Study the drawing (mm; zero at the part's minimum x, y, z) and answer. Give positions to 0.01 mm unless a question says otherwise; leave off trailing zeros. Loops run counter-clockwise (first coordinate to the right, second up) from the corner with the lowest first, then second, coordinate; pieces in that order, holes last. Notation, with made-up numbers: M 26,83.25 L 36,83.25 A13 ccw 36,107.25 Z; hole C 5,26 d6. An arc over 180 degrees is marked long. Return JSON: item names as keys, results as strings.
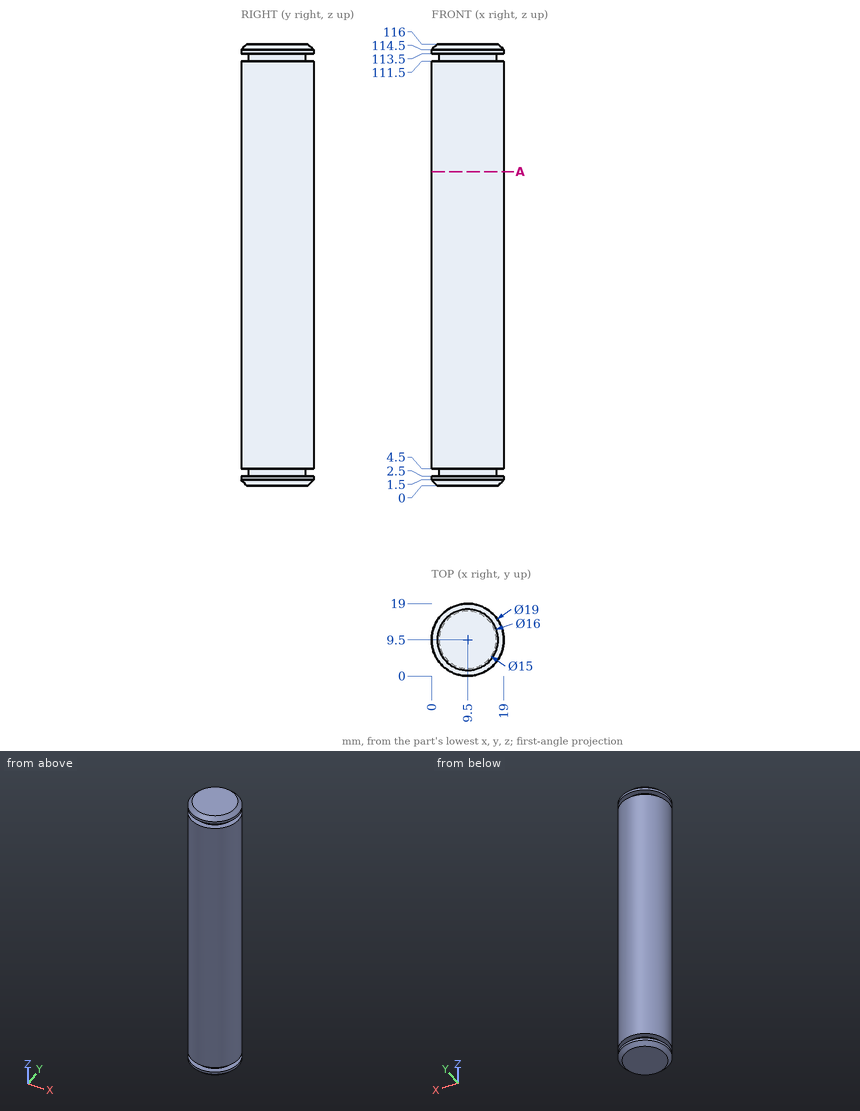
(1) Given pin 1 (10 mm diameter, centred on y = 4, z = 60.5, fed in from -X); pin 2 (1 mm diameter, centred on y = 15, z = 80, fed in from +X); pin 3 (3 mm diameter, centred on x = 14.5, z = 27, fed in from -Y), each flat-ended and moving along its own axis, determine where each tip first touches the part or whether it passes through.
Values follow:
{"pin 1": "x = 0.01", "pin 2": "x = 17.58", "pin 3": "y = 0.67"}
(2) The part is cut by section A-A (z = 82.5). Determine the outline of the cut face in (x, y), and give its area (3 significant figures).
Values follow:
{"outline": "C 9.5,9.5 d19", "area": "284 mm²"}
(3) Straight lines are drawn through the part: line 1 along Z through (x, y) = (17, 10.5); line 2 along Z through (x, y) = (15, 3); line 3 along Y through (x, z) = (10, 21). For each, find the intervals that lie inside material, in ascending order.
Values follow:
{"line 1": "0 to 2.5, 4.5 to 111.5, 113.5 to 116", "line 2": "0.51 to 2.5, 4.5 to 111.5, 113.5 to 115.49", "line 3": "0.01 to 18.99"}
